from build123d import *

# Parameters (mm, degrees)
SKETCH1_W           = 30
SKETCH1_H           = 10
SKETCH1_R           = 2.3
SKETCH1_R_2         = 1.5
BOSS_EXTRUDE1_DEPTH = 6
FILLET1_R           = 4
FILLET2_R           = 3
CUT_EXTRUDE1_REACH  = 23.433
SKETCH3_R           = 1.5
SKETCH4_R           = 1.75
CUT_EXTRUDE2_DEPTH  = 3
SKETCH7_R           = 2.5
CUT_EXTRUDE6_DEPTH  = 3
CUT_EXTRUDE7_START  = -6
SKETCH8_W           = 12
SKETCH8_H           = 1.5
CUT_EXTRUDE7_DEPTH  = 6


with BuildPart() as part:
    # Sketch1 → Boss-Extrude1 (new body)
    with BuildSketch(Plane(origin=(0, 0, 0), x_dir=(1, 0, 0), z_dir=(0, 1, 0))):
        with Locations((2.982829209, 12.310123294)):
            Rectangle(SKETCH1_W, SKETCH1_H)
        with Locations(Location((-8.017170791, 12.310123294, 0), (0, 0, 270))):
            Circle(SKETCH1_R, mode=Mode.SUBTRACT)
        with Locations(Location((13.982829209, 12.310123294, 0), (0, 0, 270))):
            Circle(SKETCH1_R_2, mode=Mode.SUBTRACT)
    extrude(amount=BOSS_EXTRUDE1_DEPTH)

    # Fillet1
    fillet1_edges = [part.edges().sort_by_distance(p)[0] for p in [
        (17.982829209, 3, -17.310123294),
        (17.982829209, 3, -7.310123294),
    ]]
    fillet(fillet1_edges, radius=FILLET1_R)

    # Fillet2
    fillet2_edges = [part.edges().sort_by_distance(p)[0] for p in [
        (-12.017170791, 3, -17.310123294),
        (-12.017170791, 3, -7.310123294),
    ]]
    fillet(fillet2_edges, radius=FILLET2_R)

    # Sketch3 → Cut-Extrude1 (cut, up to next)
    with BuildSketch(Plane(origin=(0, 0, -17.310123294), x_dir=(-1, 0, 0), z_dir=(0, 0, -1)), mode=Mode.PRIVATE) as cut_extrude1_sk1:
        with Locations((4.017170791, 3)):
            Circle(SKETCH3_R)
    cut_extrude1_tool1 = extrude(cut_extrude1_sk1.sketch, amount=-CUT_EXTRUDE1_REACH, mode=Mode.PRIVATE) & part.part
    add(cut_extrude1_tool1.solids().sort_by_distance((-4.017171, 3, -17.310123))[0], mode=Mode.SUBTRACT)

    # Sketch4 → Cut-Extrude2 (cut)
    with BuildSketch(Plane(origin=(0, 0, -17.310123294), x_dir=(-1, 0, 0), z_dir=(0, 0, -1))):
        with Locations((4.017170791, 3)):
            Circle(SKETCH4_R)
    extrude(amount=-CUT_EXTRUDE2_DEPTH, mode=Mode.SUBTRACT)

    # Sketch7 → Cut-Extrude6 (cut)
    with BuildSketch(Plane(origin=(0, 0, -17.310123294), x_dir=(-1, 0, 0), z_dir=(0, 0, -1))):
        with Locations((4.017170791, 3)):
            Circle(SKETCH7_R)
    extrude(amount=-CUT_EXTRUDE6_DEPTH, mode=Mode.SUBTRACT)

    # Sketch8 → Cut-Extrude7 (cut)
    with BuildSketch(Plane(origin=(0, 6, 0), x_dir=(1, 0, 0), z_dir=(0, 1, 0)).offset(CUT_EXTRUDE7_START)):
        with Locations((-6.017170791, 12.310123294)):
            Rectangle(SKETCH8_W, SKETCH8_H)
    extrude(amount=CUT_EXTRUDE7_DEPTH, mode=Mode.SUBTRACT)


solid = part.part
Geometry: final body of the model. Coordinates: model frame, mm. A direction names the side the tool comes from. Coordinates: 2 decimals unless noted, no trailing zeros. Order: outer loops, then holes, each group sorted by start corner. A loop starts at its lowest first (then second) coordinate and runs counter-clockwise, first axis right, second up. Notation, with made-up numbers: M 76.25,-10.75 L 126.25,-10.75 A18 cw 126.25,-2.75 Z; hole C -15.75,71 d9. An arc over 180 degrees is marked long. One line per question, with ' | ' between items. Start each with the question number.
Item 1: Pin query (flat end, axial travel): pin 1 Ø0.9 at (x, y) = (-11, 3.5) entering from -Z; pin 2 Ø0.9 at (x, y) = (-11, 1.5) entering from +Z; pin 3 Ø1.5 at (y, z) = (2.5, -14.5) entering from +X. Return the tip coordinate at first contact, or that it passes through.
Item 2: Draft query along X for faces 5 (the flat face through (-12.017, 3, -14)), 6 (the cylindrical face through (16.78, 3.04, -16.17)), 7 (the cylindrical face through (-7.98, 2.96, -14.61)), 8 (the flat face through (-2, 3, -13.06)). Return one class per face: released by +X, released by -X, zero draft, split by the parting line, or undercut.
Item 3: Cut plane B-B, the plane x = -8.5. Return the cut outline in (y, z).
Item 4: Cut plane C-C, the plane x = -4.5. Return the cut outline in (y, z).
Item 5: Cut plane A-A, the plane y = 3. Count the separate pieces of the cut face and the enclosed holes in it, then the cut area to 3 significant figures.
Item 6: Cut plane D-D, the plane z = -8.5. Return the cut outline in (x, y), then the cut area to 3 significant figures.
Item 7: Set-up query: faces 1 (the cylindrical face through (16.78, 3.04, -8.45)), 2 (the cylindrical face through (-3.48, 0.56, -15.83)), 3 (the cylindrical face through (-8.06, 2.96, -10.01)), 4 (the flat face through (-11, 3, -13.06)). Return all of +Z, -Z, +X, -X, +Y, -Y with unobstructed straight access to the full face (end or side cutting, diameter ignored); none if empty.
Item 8: Ray query, probe 1 along X at (y, z) = (2.75, -13.25); probe 2 along Z at (x, y) = (-5.25, 4.2); probe 3 along X at (y, z) = (4.5, -12.5). Return the intervals inside material, ascending. Write a range as [from, to].
A:
1) pin 1: stops at z = -16.89 | pin 2: stops at z = -7.73 | pin 3: stops at x = 17.96
2) face 5: released by -X | face 6: released by +X | face 7: undercut | face 8: zero draft
3) outline: M 0,-17.31 L 6,-17.31 L 6,-14.56 L 0,-14.56 Z; M 0,-10.06 L 6,-10.06 L 6,-7.31 L 0,-7.31 Z
4) outline: M 0,-17.31 L 0.55,-17.31 L 0.55,-14.31 L 1.58,-14.31 L 1.58,-13.06 L 0,-13.06 Z; M 0,-11.56 L 1.58,-11.56 L 1.58,-7.31 L 0,-7.31 Z; M 4.42,-14.31 L 5.45,-14.31 L 5.45,-17.31 L 6,-17.31 L 6,-13.06 L 4.42,-13.06 Z; M 4.42,-11.56 L 6,-11.56 L 6,-7.31 L 4.42,-7.31 Z
5) separate pieces: 3 | enclosed holes: 1 | area: 223 mm2
6) outline: M -11.41,0 L 16.83,0 L 16.83,6 L -11.41,6 Z; hole C -4.02,3 d3 | area: 162 mm2
7) face 1: +Z, +X, +Y, -Y | face 2: -Z | face 3: +Y, -Y | face 4: -X, +Y, -Y
8) probe 1: x = [-12.02, -10.12], [-5.92, -5.5], [-2.54, 12.81], [15.15, 17.98] | probe 2: z = [-14.31, -13.06], [-11.56, -7.31] | probe 3: x = [-0.02, 12.49], [15.47, 17.98]
